The model under review builds one solid part; all positions refer to its coordinate system, in mm. Face numbers are marked on the shaded views. A direction names the side the tool comes from. Coordinates: 2 decimals unless noted, no trailing zeros. Write each loop counter-clockwise with the first axis right and the second up, starting at its lowest first coordinate (ties: lowest second). Pieces come first, ordered by that corner, then holes. Notation, with made-up numbers: (49, 52) -> (95, 52) arc R19 ccw to (95, 77) -> close; hole circle Ø3 at (58.25, -32). An arc over 180 degrees is marked (long way). Write each question's results on one line, items separated by ' | '.
```python
from build123d import *

# Parameters (mm, degrees)
F0_W     = 450
F0_H     = 450
F1_DEPTH = 950
F2_W     = 50
F2_H     = 50
F2_W_2   = 330
F2_H_2   = 475
F3_DEPTH = 450.001
F4_W     = 380
F4_H     = 425
F5_DEPTH = 400.001
F6_W     = 380
F6_H     = 50
F6_H_2   = 252.931069
F7_DEPTH = 145.760456


with BuildPart() as f1:
    # F0 (on Top) → F1 (new body)
    with BuildSketch(Plane.XY):
        Rectangle(F0_W, F0_H)
    extrude(amount=F1_DEPTH)

    # F2 (on face) → F3 (cut, through all)
    with BuildSketch(Plane.YZ.offset(225)):
        with Locations((200, 500)):
            Rectangle(F2_W, F2_H)
        with Locations((-25, 237.5)):
            Rectangle(F2_W_2, F2_H_2)
        with Locations((200, 237.5)):
            Rectangle(F2_W, F2_H_2)
        Polygon((225, 950), (175, 525), (225, 525), align=None)
        Polygon((-225, 950), (-225, 525), (140, 525), (190, 950), align=None)
    extrude(amount=-F3_DEPTH, mode=Mode.SUBTRACT)

    # F4 (on face) → F5 (cut, through all)
    with BuildSketch(Plane(origin=(0, 175, 0), x_dir=(-1, 0, 0), z_dir=(0, 1, 0))):
        with Locations((0, 212.5)):
            Rectangle(F4_W, F4_H)
    extrude(amount=-F5_DEPTH, mode=Mode.SUBTRACT)

    # F6 (on face) → F7 (cut, through all)
    with BuildSketch(Plane(origin=(0, 77.167235, -9.078498), x_dir=(1, 0, 0), z_dir=(0, -0.993151, 0.116841))):
        with Locations((0, 865.692911)):
            Rectangle(F6_W, F6_H)
        with Locations((0, 664.227376)):
            Rectangle(F6_W, F6_H_2)
    extrude(amount=-F7_DEPTH, mode=Mode.SUBTRACT)


solid = f1.part
```
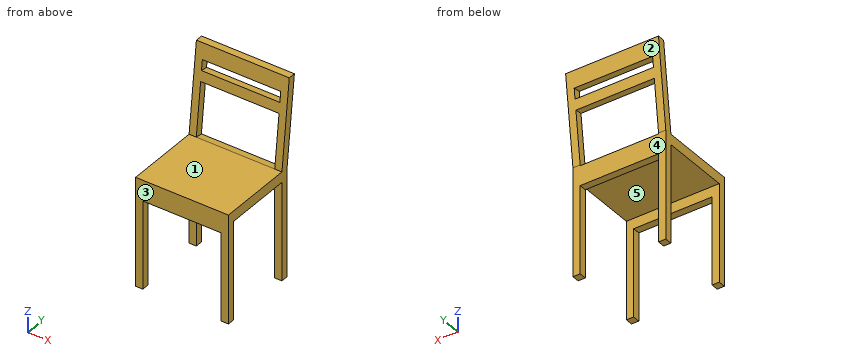
Q1. Machinability: for the marked faces 1 and 2, which of the approach directions +Z, -Z, +X, -X, +Y, -Y give a long, thin tool a straight path to every point of the face, cutting with its end or side? Answer none if there is none.
Solution:
face 1: +Z, +X, -X, -Y | face 2: -Z, +X, -X, +Y
Q2. Add section B-B (x = -85.5). Write out the cut boundary in (y, z).
Solution:
outline: (-225, 425) -> (-190, 425) -> (-190, 475) -> (140, 475) -> (140, 425) -> (175, 425) -> (175, 520.88) -> (140, 525) -> (-225, 525) -> close; (169.55, 776.2) -> (204.07, 772.14) -> (209.92, 821.79) -> (175.39, 825.86) -> close; (181.24, 875.51) -> (215.76, 871.45) -> (225, 950) -> (190, 950) -> close
Q3. Draft analysis for pull direction Y (two halves, no side actions). For the marked faces 3, 4 and 5, state which applies: pulls with the +Y half, pulls with the -Y half, needs draft (parallel to the pull), parting line crosses it, or undercut.
Solution:
face 3: pulls with the -Y half | face 4: pulls with the +Y half | face 5: undercut
Q4. Add section D-D (y = -166.5). Write out the cut boundary in (x, z).
Solution:
outline: (-225, 475) -> (225, 475) -> (225, 525) -> (-225, 525) -> close
Q5. For line 1 (Z direction, x = -158, y = -61.5); line 2 (X direction, y = 151, z = 161.5); line 3 (Z direction, x = 196, y = -192.5), list the stretches that pass through material, from the lowest coordinate up. Write a range as from..to.
Solution:
line 1: 475..525 | line 2: -225..-190, 190..225 | line 3: 0..525
Q6. Add section A-A (z = 187). Write out the cut boundary in (x, y).
Solution:
outline: (-225, -225) -> (-190, -225) -> (-190, -190) -> (-225, -190) -> close; (-225, 140) -> (-190, 140) -> (-190, 175) -> (-225, 175) -> close; (190, -225) -> (225, -225) -> (225, -190) -> (190, -190) -> close; (190, 140) -> (225, 140) -> (225, 175) -> (190, 175) -> close
Q7. Clearance check with flat-ended pins moving along their axes: P1, Ø17.5, axis at x = 65, y = -201.5, coming from the -Z side; P2, Ø2, axis at x = 92, z = 508.5, coming from the +Y side; P3, Ø6, axis at x = -47, y = -77, coming from the +Z side. State where each tip first meets the part, or that it passes through.
Solution:
P1: z = 425 | P2: y = 175 | P3: z = 525
Q8. Add section C-C (z = 635). Write out the cut boundary in (x, y), plus the area to 3 significant figures.
Solution:
outline: (-225, 152.94) -> (-190, 152.94) -> (-190, 187.94) -> (-225, 187.94) -> close; (190, 152.94) -> (225, 152.94) -> (225, 187.94) -> (190, 187.94) -> close | area: 2,450 mm²
